CAD build for the part. Positions are in the model's coordinates, mm. Face numbers are marked on the shaded views. A direction names the side the tool comes from. Give positions to 0.01 mm unless a question says otherwise; leave off trailing zeros. Write each loop counter-clockwise with the first axis right and the second up, starting at its lowest first coordinate (ties: lowest second). Pieces come first, ordered by that corner, then holes. Notation, with made-up numbers: (-37, 38.5) - (18, 38.5) arc R13 ccw to (18, 54.5) - close; hole circle Ø4 at (-23, 58). An arc over 180 degrees is marked (long way). Answer as a JSON object with one key per item and string values.
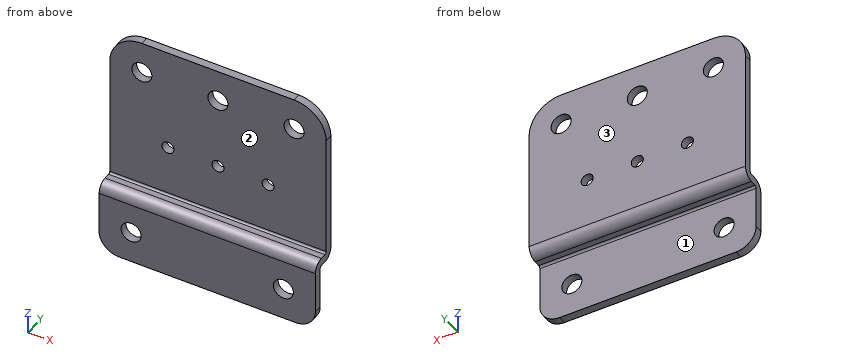
from build123d import *

# Parameters (mm, degrees)
SKETCH1_R                    = 2.5
BASE_FLANGE1_DEPTH           = 2
EDGE_FLANGE1_STRIP_W         = 9
EDGE_FLANGE1_STRIP_H         = 2
EDGE_FLANGE1_STRIP_CUT_DEPTH = 54
EDGE_FLANGE1_DEPTH           = 54
EDGE_FLANGE2_DEPTH           = 54
SKETCH25_R                   = 2.5
CUT_EXTRUDE1_DEPTH           = 69.112040052
SKETCH26_R                   = 1.5
CUT_EXTRUDE2_DEPTH           = 2


# Sheet-metal steps are written as plain solids
with BuildPart() as part:
    # Sketch1 → Base-Flange1 (new body)
    with BuildSketch(Plane(origin=(0, 0, 0), x_dir=(1, 0, 0), z_dir=(0, 1, 0))):
        with BuildLine():
            Line((0, 0), (54, 0))
            Line((54, 0), (54, 11))
            ThreePointArc((54, 11), (52.535533906, 14.535533906), (49, 16))
            Line((49, 16), (5, 16))
            ThreePointArc((5, 16), (1.464466094, 14.535533906), (0, 11))
            Line((0, 11), (0, 0))
        make_face()
        with Locations(Location((8, 8, 0), (0, 0, 270))):
            Circle(SKETCH1_R, mode=Mode.SUBTRACT)
        with Locations(Location((46, 8, 0), (0, 0, 90))):
            Circle(SKETCH1_R, mode=Mode.SUBTRACT)
    extrude(amount=-BASE_FLANGE1_DEPTH)

    # Edge-Flange1 strip (across the edge) → Edge-Flange1 strip cut (cut)
    with BuildSketch(Plane(origin=(0, 0, 0), x_dir=(0, 0, -1), z_dir=(1, 0, 0))):
        with Locations((-4, -1)):
            Rectangle(EDGE_FLANGE1_STRIP_W, EDGE_FLANGE1_STRIP_H)
    extrude(amount=EDGE_FLANGE1_STRIP_CUT_DEPTH, mode=Mode.SUBTRACT)

    # Edge-Flange1 section (across the edge) → Edge-Flange1 (add)
    with BuildSketch(Plane(origin=(0, 0, 0), x_dir=(0, 0, -1), z_dir=(1, 0, 0))):
        with BuildLine():
            Line((-2, 0.5), (-2, 2))
            Line((-2, 2), (0, 2))
            Line((0, 2), (0, 0.5))
            ThreePointArc((0, 0.5), (0.146446609, 0.146446609), (0.5, 0))
            Line((0.5, 0), (0.5, -2))
            ThreePointArc((0.5, -2), (-1.267766953, -1.267766953), (-2, 0.5))
        make_face()
    extrude(amount=EDGE_FLANGE1_DEPTH)

    # Edge-Flange2 section (across the edge) → Edge-Flange2 (add)
    with BuildSketch(Plane(origin=(54, 2.5, 2), x_dir=(0, -1, 0), z_dir=(-1, 0, 0))):
        with BuildLine():
            Line((-2, 0.5), (-2, 39))
            Line((-2, 39), (0, 39))
            Line((0, 39), (0, 0.5))
            ThreePointArc((0, 0.5), (0.146446609, 0.146446609), (0.5, 0))
            Line((0.5, 0), (0.5, -2))
            ThreePointArc((0.5, -2), (-1.267766953, -1.267766953), (-2, 0.5))
        make_face()
    extrude(amount=EDGE_FLANGE2_DEPTH)

    # Sketch25 → Cut-Extrude1 (cut, through all)
    with BuildSketch(Plane(origin=(0, 4.5, 0), x_dir=(1, 0, 0), z_dir=(0, 1, 0))):
        with Locations(Location((27, -33, 0), (0, 0, 270))):
            Circle(SKETCH25_R)
        with Locations(Location((8, -33, 0), (0, 0, 270))):
            Circle(SKETCH25_R)
        with BuildLine():
            ThreePointArc((8, -41), (2.343145751, -38.656854249), (0, -33))
            Line((0, -33), (0, -41))
            Line((0, -41), (8, -41))
        make_face()
        with Locations(Location((46, -33, 0), (0, 0, 270))):
            Circle(SKETCH25_R)
        with BuildLine():
            Line((54, -41), (54, -33))
            ThreePointArc((54, -33), (51.656854249, -38.656854249), (46, -41))
            Line((46, -41), (54, -41))
        make_face()
    extrude(amount=-CUT_EXTRUDE1_DEPTH, mode=Mode.SUBTRACT)

    # Sketch26 → Cut-Extrude2 (cut)
    with BuildSketch(Plane(origin=(0, 4.5, 0), x_dir=(1, 0, 0), z_dir=(0, 1, 0))):
        with Locations(Location((39.5, -14.92, 0), (0, 0, 270))):
            Circle(SKETCH26_R)
        with Locations(Location((27, -14.92, 0), (0, 0, 270))):
            Circle(SKETCH26_R)
        with Locations(Location((14.5, -14.92, 0), (0, 0, 270))):
            Circle(SKETCH26_R)
    extrude(amount=-CUT_EXTRUDE2_DEPTH, mode=Mode.SUBTRACT)


solid = part.part
Item 1: Probe line 1 (X direction, y = -1.5, z = -8); line 2 (X direction, y = 3.05, z = 14.92); line 3 (X direction, y = 3.95, z = 33). List the from-to ranges inside material, lowest first. Write a range as from..to.
Entries:
{"line 1": "0..5.5, 10.5..43.5, 48.5..54", "line 2": "0..13, 16..25.5, 28.5..38, 41..54", "line 3": "0..5.5, 10.5..24.5, 29.5..43.5, 48.5..54"}
Item 2: Flat gauge pins, fed straight in: P1, Ø8, axis at x = 25, z = -10, coming from the +Y side; P2, Ø4, axis at x = 48, z = 12.5, coming from the -Y side; P3, Ø1.6, axis at x = 27, y = 1, coming from the -Z side. Where does each tip first touch, or does it go through?
Entries:
{"P1": "y = 0", "P2": "y = 2.5", "P3": "z = -0.1"}
Item 3: Cut at B-B (x = 27). Give the cut face in (y, z).
Entries:
{"outline": "(-2, -16) - (0, -16) - (0, -0.5) arc R0.5 cw to (0.5, 0) - (2, 0) arc R2.5 ccw to (4.5, 2.5) - (4.5, 13.42) - (2.5, 13.42) - (2.5, 2.5) arc R0.5 cw to (2, 2) - (0.5, 2) arc R2.5 ccw to (-2, -0.5) - close; (2.5, 16.42) - (4.5, 16.42) - (4.5, 30.5) - (2.5, 30.5) - close; (2.5, 35.5) - (4.5, 35.5) - (4.5, 41) - (2.5, 41) - close"}
Item 4: Which spindle directions (+Z, -Z, +X, -X, +Y, -Y) get a long thin tool onto all of the face, cutting with end or side? Do the marked faces 1, 2 and 3. Say none if no direction does.
Entries:
{"face 1": "-Z, +X, -X, +Y", "face 2": "+Z, +X, -X, -Y", "face 3": "+Z, -Z, +X, -X, +Y"}
Item 5: Cut at D-D (z = 14.92). Give the cut face in (x, y).
Entries:
{"outline": "(0, 2.5) - (13, 2.5) - (13, 4.5) - (0, 4.5) - close; (16, 2.5) - (25.5, 2.5) - (25.5, 4.5) - (16, 4.5) - close; (28.5, 2.5) - (38, 2.5) - (38, 4.5) - (28.5, 4.5) - close; (41, 2.5) - (54, 2.5) - (54, 4.5) - (41, 4.5) - close"}
Item 6: Cut at C-C (y = 3.5). Give the cut face in (x, z), and give its area (3 significant figures).
Entries:
{"outline": "(0, 0.5) - (54, 0.5) - (54, 33) arc R8 ccw to (46, 41) - (8, 41) arc R8 ccw to (0, 33) - close; hole circle Ø5 at (8, 33); hole circle Ø3 at (14.5, 14.92); hole circle Ø5 at (27, 33); hole circle Ø3 at (27, 14.92); hole circle Ø3 at (39.5, 14.92); hole circle Ø5 at (46, 33)", "area": "2,080 mm2"}
Item 7: Cut at A-A (z = -8). Give the cut face in (x, y).
Entries:
{"outline": "(0, -2) - (5.5, -2) - (5.5, 0) - (0, 0) - close; (10.5, -2) - (43.5, -2) - (43.5, 0) - (10.5, 0) - close; (48.5, -2) - (54, -2) - (54, 0) - (48.5, 0) - close"}
